from build123d import *

# Parameters (mm, degrees)
CUT_EXTRUDE1_START = 25.65654
CUT_EXTRUDE1_DEPTH = 2.802619264


with BuildPart() as part:
    # Sketch2 → Revolve1 (revolve)
    with BuildSketch(Plane(origin=(0, 0, 0), x_dir=(0, 0, -1), z_dir=(1, 0, 0)), mode=Mode.PRIVATE) as revolve1_sk:
        with BuildLine():
            Line((-26.6827, 1.5875), (-26.6827, 2.2225))
            ThreePointArc((-26.6827, 2.2225), (-25.767752118, 3.57733025), (-24.480157143, 4.5847))
            Line((-24.480157143, 4.5847), (-24.1173, 4.5847))
            Line((-24.1173, 4.5847), (-24.1173, 2.413))
            Line((-24.1173, 2.413), (26.0873875, 2.413))
            Line((26.0873875, 2.413), (26.6827, 1.8176875))
            Line((26.6827, 1.8176875), (26.6827, 0))
            Line((26.6827, 0), (-24.739996448, 0))
            Line((-24.739996448, 0), (-25.65654, 1.5875))
            Line((-25.65654, 1.5875), (-26.6827, 1.5875))
        make_face()
    revolve(revolve1_sk.sketch.rotate(Axis((0, 0, 26.6827), (0, 0, -1)), 90), axis=Axis((0, 0, 26.6827), (0, 0, -1)))

    # Sketch3 → Cut-Extrude1 (cut, through all)
    with BuildSketch(Plane.XY.offset(CUT_EXTRUDE1_START)):
        Polygon((0, 1.833087105), (-1.5875, 0.916543552), (-1.5875, -0.916543552), (0, -1.833087105), (1.5875, -0.916543552), (1.5875, 0.916543552), align=None)
    extrude(amount=CUT_EXTRUDE1_DEPTH, mode=Mode.SUBTRACT)


solid = part.part
Model file for the job. Use its own axes, mm. A direction names the side the tool comes from. Give positions to 0.01 mm unless a question says otherwise; leave off trailing zeros. Loops run counter-clockwise (first coordinate to the right, second up) from the corner with the lowest first, then second, coordinate; pieces in that order, holes last.
Item 1: Which spindle directions (+Z, -Z, +X, -X, +Y, -Y) get a long thin tool onto all of the face, cutting with end or side? Do faces 4 (the face through (-1.915, 1.468, -1.336)), 5 (the face through (1.588, 0, 26)), 6 (the face through (-2, 0, 26.683)). Say none if no direction does.
Check values:
face 4: -Z
face 5: +Z
face 6: +Z, +X, -X, +Y, -Y
Item 2: Slice it at C-C (y = -4). Write the cut outline in (x, z), plus the area to 3 significant figures.
Check values:
outline: (-2.24, 24.12) - (2.24, 24.12) - (2.24, 24.48) arc R3.39 ccw to (-2.24, 24.48) - close
area: 4.22 mm2
Item 3: Slice it at B-B (x = -3). Write the cut outline in (y, z), plus the area to 3 significant figures.
Check values:
outline: (-3.47, 24.12) - (3.47, 24.12) - (3.47, 24.48) arc R4.3 ccw to (-3.47, 24.48) - close
area: 11.0 mm2
Item 4: Drop flat-ended pins along their axis: P1, Ø1, axis at x = 2.5, z = 16.5, coming from the -Y side; P2, Ø3, axis at y = -1, z = 9, coming from the -X side; P3, Ø5, axis at x = 2.5, z = 18.5, coming from the -Y side; P4, Ø0.6, axis at x = -1, y = 1, coming from the +Z side. Give the stop position or say it passes through.
Check values:
P1: stops at y = -1.35
P2: stops at x = -2.41
P3: stops at y = -2.41
P4: stops at z = 26.68
Item 5: Slice it at A-A (z = 21). Write the cut outline in (x, y).
Check values:
outline: circle Ø4.83 at (0, 0)
Item 6: Mould opens along X. For faces 1 (the face through (-1.588, 0, 26)), 2 (the face through (-0.994, 4.476, 24.296)), 3 (the face through (0, 0, -26.683)) say: +X half, -X half, draft (parallel to the pull), parting line (faces both ways), or undercut.
Check values:
face 1: undercut
face 2: parting line
face 3: draft
Item 7: Drill centre lines: line 1 along X through (y, z) = (0.75, -3); line 2 along Z through (x, y) = (2.5, -0.5); line 3 along Z through (x, y) = (0.5, 1.75). Where is each one in solid material? Low to high.
Check values:
line 1: x = -2.29 to 2.29
line 2: z = 24.12 to 26.52
line 3: z = -26.68 to 26.68
